from build123d import *

# Parameters (mm, degrees)
F0_W      = 1352.55
F0_H      = 514.35
F1_DEPTH  = 25.4
F2_W      = 50.8
F2_H      = 317.5
F3_DEPTH  = 38.1
F4_W      = 50.8
F4_H      = 76.2
F5_DEPTH  = 660.4
F6_W      = 50.8
F6_H      = 508
F7_DEPTH  = 25.4
F8_R      = 25.4
F9_R      = 25.39999
F10_R     = 25.4
F11_R     = 25.39999
F12_R     = 25.39999
F13_R     = 25.39999
F14_W     = 1201.120785141
F14_H     = 25.4
F15_DEPTH = 304.8


# Not quite as in the source:
# - a fillet or chamfer is up to 0.001 mm smaller than in the source, because OpenCascade refuses the exact size


with BuildPart() as f1:
    # F0 (on Top) → F1 (new body)
    with BuildSketch(Plane.XY):
        with Locations((3.3097676933, -84.2684167102)):
            Rectangle(F0_W, F0_H)
    extrude(amount=F1_DEPTH)

    # F2 (on face) → F3 (join)
    with BuildSketch(Plane.XY.offset(25.4)):
        with Locations((-625.9603925705, -81.0934167102)):
            Rectangle(F2_W, F2_H)
        with Locations((625.9603925705, -81.0934167102)):
            Rectangle(F2_W, F2_H)
    extrude(amount=-F3_DEPTH)

    # F4 (on face) → F5 (join)
    with BuildSketch(Plane(origin=(0, 0, 0), x_dir=(1, 0, 0), z_dir=(0, 0, -1))):
        with Locations((-625.9603925705, 277.9434167102)):
            Rectangle(F4_W, F4_H)
        with Locations((625.9603925705, 277.9434167102)):
            Rectangle(F4_W, F4_H)
    extrude(amount=F5_DEPTH)

    # F6 (on face) → F7 (join)
    with BuildSketch(Plane(origin=(0, 0, -660.4), x_dir=(1, 0, 0), z_dir=(0, 0, -1))):
        with Locations((625.9603925705, 122.6374032485)):
            Rectangle(F6_W, F6_H)
        with Locations((-625.9603925705, 122.6374032485)):
            Rectangle(F6_W, F6_H)
    extrude(amount=F7_DEPTH)

    # F8
    f8_edges = [f1.edges().sort_by_distance(p)[0] for p in [
        (651.360393, 131.362597, -673.1),
    ]]
    fillet(f8_edges, radius=F8_R)

    # F9 (radius 25.4 in the source; OpenCascade refuses exactly that, so slightly less here)
    f9_edges = [f1.edges().sort_by_distance(p)[0] for p in [
        (600.560393, 131.362597, -673.1),
    ]]
    fillet(f9_edges, radius=F9_R)

    # F10
    f10_edges = [f1.edges().sort_by_distance(p)[0] for p in [
        (651.360393, -376.637403, -673.1),
    ]]
    fillet(f10_edges, radius=F10_R)

    # F11 (radius 25.4 in the source; OpenCascade refuses exactly that, so slightly less here)
    f11_edges = [f1.edges().sort_by_distance(p)[0] for p in [
        (600.560393, -376.637403, -673.1),
    ]]
    fillet(f11_edges, radius=F11_R)

    # F12 (radius 25.4 in the source; OpenCascade refuses exactly that, so slightly less here)
    f12_edges = [f1.edges().sort_by_distance(p)[0] for p in [
        (-600.560393, -376.637403, -673.1),
        (-651.360393, -376.637403, -673.1),
    ]]
    fillet(f12_edges, radius=F12_R)

    # F13 (radius 25.4 in the source; OpenCascade refuses exactly that, so slightly less here)
    f13_edges = [f1.edges().sort_by_distance(p)[0] for p in [
        (-651.360393, 131.362597, -673.1),
        (-600.560393, 131.362597, -673.1),
    ]]
    fillet(f13_edges, radius=F13_R)

    # F14 (on face) → F15 (join)
    with BuildSketch(Plane(origin=(0, 0, 0), x_dir=(1, 0, 0), z_dir=(0, 0, -1))):
        with Locations((0, 303.3434167102)):
            Rectangle(F14_W, F14_H)
    extrude(amount=F15_DEPTH)


solid = f1.part
Geometry check sheet. Reference: the model listing, model coordinates, mm. A direction names the side the tool comes from. Round coordinates to 2 decimals unless told otherwise and drop trailing zeros. Loops run counter-clockwise (first coordinate to the right, second up) from the corner with the lowest first, then second, coordinate; pieces in that order, holes last. Notation, with made-up numbers: (57.5, -20.75) -> (81.5, -20.75) arc R10 cw to (81.5, -1.75) -> close; hole circle Ø9 at (62, -29.5). An arc over 180 degrees is marked (long way). Answer as a JSON object with one key per item and string values. Group by question number.
Item 1: Release check for a two-part mould opening along X. For faces 1 (the face through (-607.803, -368.999, -673.278)), 2 (the face through (-644.117, -368.999, -673.278)), 3 (the face through (-626, -57, -660.4)) record: pulls with the +X half, pulls with the -X half, needs draft (parallel to the pull), parting line crosses it, or undercut.
Item 2: Cross-section at B-B, the plane z = -347. Record the cut outline in (x, y), plus the area to 3 significant figures.
Item 3: Thickness scan on line 1 along X through (y, z) = (-286.5, -509.5); line 2 along Z through (x, y) = (-566, -119.5); line 3 along Y through (x, z) = (605, -492). Record the ranges inside material, lowest first.
Item 4: Set-up check for faces 4 (the face through (626, -57, -660.4)), 5 (the face through (-626, -347, -660.4)), 6 (the face through (-8, -304, -304.8)), 7 (the face through (-600.56, -240, -367)): record each of +Z, -Z, +X, -X, +Y, -Y from which the full face is reachable in a straight line by a thin tool's end or side.
Item 5: Depth check by flat-ended pin: pin 1 Ø12.5 at (x, y) = (18, -302.5) entering from -Z; pin 2 Ø1 at (x, y) = (-228, 103.5) entering from -Z. Enter the tip coordinate at first touch or a pass-through.
Item 6: Cross-section at D-D, the plane x = 415. Record the cut outline in (y, z), plus the area to 3 significant figures.
Item 7: Cross-section at C-C, the plane z = -44. Record the cut outline in (x, y), plus the area to 3 significant figures.
Item 8: Cross-section at A-A, the plane y = 10. Record the cut outline in (x, z), plus the area to 3 significant figures.
Determined:
{
 "1": {"face 1": "undercut", "face 2": "pulls with the -X half", "face 3": "needs draft"},
 "2": {"outline": "(-651.36, -316.04) -> (-600.56, -316.04) -> (-600.56, -239.84) -> (-651.36, -239.84) -> close; (600.56, -316.04) -> (651.36, -316.04) -> (651.36, -239.84) -> (600.56, -239.84) -> close", "area": "7,740 mm²"},
 "3": {"line 1": "x = -651.36 to -600.56, 600.56 to 651.36", "line 2": "z = 0 to 25.4", "line 3": "y = -316.04 to -239.84"},
 "4": {"face 4": "+X, -X, +Y", "face 5": "+X, -X, -Y", "face 6": "-Z, +Y, -Y", "face 7": "-Z, +Y"},
 "5": {"pin 1": "stops at z = -304.8", "pin 2": "stops at z = 0"},
 "6": {"outline": "(-341.44, 0) -> (-316.04, 0) -> (-316.04, -304.8) -> (-290.64, -304.8) -> (-290.64, 0) -> (172.91, 0) -> (172.91, 25.4) -> (-341.44, 25.4) -> close", "area": "20,800 mm²"},
 "7": {"outline": "(-651.36, -316.04) -> (651.36, -316.04) -> (651.36, -239.84) -> (600.56, -239.84) -> (600.56, -290.64) -> (-600.56, -290.64) -> (-600.56, -239.84) -> (-651.36, -239.84) -> close", "area": "38,300 mm²"},
 "8": {"outline": "(-672.97, 0) -> (-651.36, 0) -> (-651.36, -12.7) -> (-600.56, -12.7) -> (-600.56, 0) -> (600.56, 0) -> (600.56, -12.7) -> (651.36, -12.7) -> (651.36, 0) -> (679.58, 0) -> (679.58, 25.4) -> (-672.97, 25.4) -> close; (-651.36, -685.8) -> (-600.56, -685.8) -> (-600.56, -660.4) -> (-651.36, -660.4) -> close; (600.56, -685.8) -> (651.36, -685.8) -> (651.36, -660.4) -> (600.56, -660.4) -> close", "area": "38,200 mm²"}
}
